Check sheet for the modelled part. Datum: model origin and axes. Units: mm. A direction names the side the tool comes from. Give positions to 0.01 mm unless a question says otherwise; leave off trailing zeros. Write each loop counter-clockwise with the first axis right and the second up, starting at its lowest first coordinate (ties: lowest second). Pieces come first, ordered by that corner, then holes. Notation, with made-up numbers: (50.5, 8) -> (72.5, 8) arc R18 cw to (72.5, 43) -> close; hole circle Ø4 at (11, -22). An arc over 180 degrees is marked (long way). Answer as a JSON object with one key per item and string values.
from build123d import *

# Parameters (mm, degrees)
EXTRUDE_1_DEPTH          = 22.5
CUT_EXTRUDE_1_DEPTH      = 55
CUT_EXTRUDE_1_DEPTH_BACK = 117
SKETCH_2_R               = 1.1
SKETCH_5_W               = 13
SKETCH_5_H               = 5
EXTRUDE_4_DEPTH          = 58
CHAMFER_1_SIZE           = 5
SKETCH_6_W               = 10.28735427
SKETCH_6_H               = 3.2
SKETCH_6_W_2             = 10.2120241
EXTRUDE_5_DEPTH          = 27
CUT_EXTRUDE_2_DEPTH      = 27
SKETCH_8_R               = 1.65
CUT_EXTRUDE_3_DEPTH      = 27
SKETCH_11_W              = 10
SKETCH_11_H              = 23.011480114
EXTRUDE_6_DEPTH          = 22.5
SKETCH_12_W              = 5
SKETCH_12_H              = 22.5
CUT_EXTRUDE_5_DEPTH      = 22
EXTRUDE_8_DEPTH          = 22
SKETCH_16_W              = 2.5
SKETCH_16_H              = 22.5
EXTRUDE_9_DEPTH          = 6
SKETCH_17_R              = 1.65
CUT_EXTRUDE_7_DEPTH      = 14


with BuildPart() as part:
    # 草图1 → 凸台-拉伸1 (new body)
    with BuildSketch(Plane(origin=(0, 0, 0), x_dir=(1, 0, 0), z_dir=(0, 1, 0))):
        Polygon((40.1, -19.5), (40.1, 11.5), (35.1, 11.5), (35.1, -11.5), (-35.1, -11.5), (-35.1, 11.5), (-40.1, 11.5), (-40.1, -19.5), align=None)
    extrude(amount=EXTRUDE_1_DEPTH)

    # 草图2 → 切除-拉伸1 (cut, two sides: drawn at the far end of the back side and taken through both)
    with BuildSketch(Plane.ZY.offset(40.1).offset(-CUT_EXTRUDE_1_DEPTH_BACK)):
        with Locations(Location((-8.5, 15.5, 0), (0, 0, 180))):
            Circle(SKETCH_2_R)
        with Locations(Location((3.5, 15.5, 0), (0, 0, 180))):
            Circle(SKETCH_2_R)
        with Locations(Location((3.5, 7.5, 0), (0, 0, 180))):
            Circle(SKETCH_2_R)
        with Locations(Location((-8.5, 7.5, 0), (0, 0, 180))):
            Circle(SKETCH_2_R)
    extrude(amount=CUT_EXTRUDE_1_DEPTH + CUT_EXTRUDE_1_DEPTH_BACK, mode=Mode.SUBTRACT)

    # 草图5 → 凸台-拉伸4 (add)
    with BuildSketch(Plane(origin=(40.1, 0, 0), x_dir=(0, 0, -1), z_dir=(1, 0, 0))):
        with Locations((-13, 5.25)):
            Rectangle(SKETCH_5_W, SKETCH_5_H)
    extrude(amount=EXTRUDE_4_DEPTH)

    # 倒角1
    chamfer_1_edges = [part.edges().sort_by_distance(p)[0] for p in [
        (40.1, 7.75, 13),
    ]]
    chamfer(chamfer_1_edges, length=CHAMFER_1_SIZE)

    # 草图6 → 凸台-拉伸5 (add)
    with BuildSketch(Plane.XZ.offset(-2.75)):
        with Locations((41.744298765, 8.1)):
            Rectangle(SKETCH_6_W, SKETCH_6_H)
        with Locations((92.99398795, 8.1)):
            Rectangle(SKETCH_6_W_2, SKETCH_6_H)
    extrude(amount=EXTRUDE_5_DEPTH)

    # 草图7 → 切除-拉伸2 (cut)
    with BuildSketch(Plane.XY.offset(9.7)):
        with BuildLine():
            Line((89.983046701, -13.162177047), (89.983046701, -0.162177047))
            ThreePointArc((89.983046701, -0.162177047), (91.583046701, 1.437822953), (93.183046701, -0.162177047))
            Line((93.183046701, -0.162177047), (93.183046701, -13.162177047))
            ThreePointArc((93.183046701, -13.162177047), (91.583046701, -14.762177047), (89.983046701, -13.162177047))
        make_face()
        with BuildLine():
            Line((41.3879759, -13.162177047), (41.3879759, -0.162177047))
            ThreePointArc((41.3879759, -0.162177047), (42.9879759, 1.437822953), (44.5879759, -0.162177047))
            Line((44.5879759, -0.162177047), (44.5879759, -13.162177047))
            ThreePointArc((44.5879759, -13.162177047), (42.9879759, -14.762177047), (41.3879759, -13.162177047))
        make_face()
    extrude(amount=-CUT_EXTRUDE_2_DEPTH, mode=Mode.SUBTRACT)

    # 草图8 → 切除-拉伸3 (cut)
    with BuildSketch(Plane.XY.offset(9.7)):
        with Locations((92.99398795, -20.25)):
            Circle(SKETCH_8_R)
        with Locations((42.99398795, -20.25)):
            Circle(SKETCH_8_R)
    extrude(amount=-CUT_EXTRUDE_3_DEPTH, mode=Mode.SUBTRACT)

    # 草图11 → 凸台-拉伸6 (add)
    with BuildSketch(Plane.XZ):
        with Locations((-6, -0.005740057)):
            Rectangle(SKETCH_11_W, SKETCH_11_H)
    extrude(amount=-EXTRUDE_6_DEPTH)

    # 草图12 → 切除-拉伸5 (cut)
    with BuildSketch(Plane(origin=(0, 0, -11.511480114), x_dir=(-1, 0, 0), z_dir=(0, 0, -1))):
        with Locations((6, 11.25)):
            Rectangle(SKETCH_12_W, SKETCH_12_H)
    extrude(amount=-CUT_EXTRUDE_5_DEPTH, mode=Mode.SUBTRACT)

    # 草图14 → 凸台-拉伸8 (add)
    with BuildSketch(Plane(origin=(0, 0, -11.511480114), x_dir=(-1, 0, 0), z_dir=(0, 0, -1))):
        with BuildLine():
            ThreePointArc((8.5, 2.276960614), (7.361519693, 1.138480307), (8.5, 0))
            Line((8.5, 0), (8.5, 2.276960614))
        make_face()
        with BuildLine():
            ThreePointArc((8.5, 5.276960614), (7.361519693, 4.138480307), (8.5, 3))
            Line((8.5, 3), (8.5, 5.276960614))
        make_face()
        with BuildLine():
            ThreePointArc((8.5, 8.276960614), (7.361519693, 7.138480307), (8.5, 6))
            Line((8.5, 6), (8.5, 8.276960614))
        make_face()
        with BuildLine():
            ThreePointArc((8.5, 11.276960614), (7.361519693, 10.138480307), (8.5, 9))
            Line((8.5, 9), (8.5, 11.276960614))
        make_face()
        with BuildLine():
            ThreePointArc((8.5, 17.276960614), (7.361519693, 16.138480307), (8.5, 15))
            Line((8.5, 15), (8.5, 17.276960614))
        make_face()
        with BuildLine():
            ThreePointArc((8.5, 20.276960614), (7.361519693, 19.138480307), (8.5, 18))
            Line((8.5, 18), (8.5, 20.276960614))
        make_face()
        with BuildLine():
            ThreePointArc((8.5, 14.276960614), (7.361519693, 13.138480307), (8.5, 12))
            Line((8.5, 12), (8.5, 14.276960614))
        make_face()
    extrude(amount=-EXTRUDE_8_DEPTH)

    # 草图16 → 凸台-拉伸9 (add)
    with BuildSketch(Plane(origin=(0, 0, -11.511480114), x_dir=(-1, 0, 0), z_dir=(0, 0, -1))):
        with Locations((9.75, 11.25)):
            Rectangle(SKETCH_16_W, SKETCH_16_H)
        with Locations((2.25, 11.25)):
            Rectangle(SKETCH_16_W, SKETCH_16_H)
    extrude(amount=EXTRUDE_9_DEPTH)

    # 草图17 → 切除-拉伸7 (cut)
    with BuildSketch(Plane.ZY.offset(11)):
        with Locations(Location((-14.289107962, 4.226014106, 0), (0, 0, 180))):
            Circle(SKETCH_17_R)
        with Locations(Location((-14.289107962, 16.747856376, 0), (0, 0, 180))):
            Circle(SKETCH_17_R)
    extrude(amount=-CUT_EXTRUDE_7_DEPTH, mode=Mode.SUBTRACT)


solid = part.part
1. Go/stop test with flat-tipped pins: P1, Ø2.5, axis at y = 4.23, z = -14.29, coming from the -X side; P2, Ø1.6, axis at y = -9.5, z = 8, coming from the -X side; P3, Ø4, axis at x = -7.5, z = -7.5, coming from the +Y side; P4, Ø8, axis at x = 53.5, z = 8.5, coming from the -Y side. Record where each tip stops, or that it passes through.
Determined:
{"P1": "through", "P2": "x = 36.6", "P3": "y = 22.5", "P4": "y = 2.75"}
2. Sectioned sample at A-A, the plane y = -1.5. Enter the section's corners in (x, z).
Determined:
{"outline": "(36.6, 6.5) -> (41.39, 6.5) -> (41.39, 9.7) -> (36.6, 9.7) -> close; (44.59, 6.5) -> (46.89, 6.5) -> (46.89, 9.7) -> (44.59, 9.7) -> close; (87.89, 6.5) -> (89.98, 6.5) -> (89.98, 9.7) -> (87.89, 9.7) -> close; (93.18, 6.5) -> (98.1, 6.5) -> (98.1, 9.7) -> (93.18, 9.7) -> close"}
3. Sectioned sample at D-D, the plane x = 9.5. Enter the section's corners in (y, z), plus the area to 3 significant figures.
Determined:
{"outline": "(0, 11.5) -> (22.5, 11.5) -> (22.5, 19.5) -> (0, 19.5) -> close", "area": "180 mm^2"}
4. Sectioned sample at C-C, the plane y = -20.25. Enter the section's corners in (x, z), plus the area to 3 significant figures.
Determined:
{"outline": "(36.6, 6.5) -> (41.34, 6.5) -> (41.34, 9.7) -> (36.6, 9.7) -> close; (44.64, 6.5) -> (46.89, 6.5) -> (46.89, 9.7) -> (44.64, 9.7) -> close; (87.89, 6.5) -> (91.34, 6.5) -> (91.34, 9.7) -> (87.89, 9.7) -> close; (94.64, 6.5) -> (98.1, 6.5) -> (98.1, 9.7) -> (94.64, 9.7) -> close", "area": "44.5 mm^2"}
5. Scan lines: L1, parallel to X at y = 1, z = 11; L2, parallel to X at y = -20, z = 7; L3, parallel to Y at x = 37.85, z = -8.5. Record each from-to range of solid material in increasing order. Write a range as [from, to].
Determined:
{"L1": "[-40.1, -35.1], [-11, -1], [35.1, 40.1]", "L2": "[36.6, 41.36], [44.62, 46.89], [87.89, 91.36], [94.62, 98.1]", "L3": "[0, 6.4], [8.6, 14.4], [16.6, 22.5]"}
6. Sectioned sample at B-B, the plane z = -6. State how many separate pieces and enclosed holes the cut face has, plus the area to 3 significant figures.
Determined:
{"separate pieces": "4", "enclosed holes": "0", "area": "352 mm^2"}
7. Access from +Z, -Z, +X, -X, +Y, -Y to the whole of each face (thin tool, end or side, straight path). Record for faces 4 (the face through (35.1, 11, 0)), 5 (the face through (-7.36, 1.16, -0.67)), 6 (the face through (69, 2.75, 13)).
Determined:
{"face 4": "-Z, +Y, -Y", "face 5": "-Z", "face 6": "+Z, -Y"}
8. Mould release check, pull along Z, two halves, no side actions. Record for faces 1 (the face through (-9.768, 4.858, -15.813)), 2 (the face through (38, 11, -11.5)), 3 (the face through (-11, 11, -3)): released by +Z, released by -Z, zero draft, split by the parting line, or undercut.
Determined:
{"face 1": "undercut", "face 2": "released by -Z", "face 3": "zero draft"}
